```python
from build123d import *

# Parameters (mm, degrees)
SKETCH1_R           = 29
BOSS_EXTRUDE1_DEPTH = 30
SKETCH2_OUTSIDE_W   = 77.468
SKETCH2_OUTSIDE_H   = 77.468
SKETCH2_OUTSIDE_R   = 23
CUT_EXTRUDE1_DEPTH  = 22
CHAMFER1_SIZE       = 6
CHAMFER1_SIZE2      = 5.034597787
SKETCH3_R           = 25
BOSS_EXTRUDE2_DEPTH = 20
SKETCH4_R           = 5
BOSS_EXTRUDE3_DEPTH = 20
CHAMFER2_SIZE       = 2


with BuildPart() as part:
    # Sketch1 → Boss-Extrude1 (new body)
    with BuildSketch(Plane.XY):
        Circle(SKETCH1_R)
    extrude(amount=BOSS_EXTRUDE1_DEPTH)

    # Sketch2 outside → Cut-Extrude1 (cut)
    with BuildSketch(Plane.XY.offset(30)):
        Rectangle(SKETCH2_OUTSIDE_W, SKETCH2_OUTSIDE_H)
        Circle(SKETCH2_OUTSIDE_R, mode=Mode.SUBTRACT)
    extrude(amount=-CUT_EXTRUDE1_DEPTH, mode=Mode.SUBTRACT)

    # Chamfer1
    chamfer1_edges = [part.edges().sort_by_distance(p)[0] for p in [
        (-29, 0, 8),
    ]]
    chamfer1_side = [part.faces().sort_by_distance(p)[0] for p in [
        (-29, 0, 4),
    ]]
    chamfer(chamfer1_edges, length=CHAMFER1_SIZE, length2=CHAMFER1_SIZE2, reference=chamfer1_side[0])

    # Sketch3 → Boss-Extrude2 (add)
    with BuildSketch(Plane.XY.offset(30)):
        Circle(SKETCH3_R)
    extrude(amount=BOSS_EXTRUDE2_DEPTH)

    # Sketch4 → Boss-Extrude3 (add)
    with BuildSketch(Plane(origin=(0, 0, 0), x_dir=(-1, 0, 0), z_dir=(0, 0, -1))):
        Circle(SKETCH4_R)
    extrude(amount=BOSS_EXTRUDE3_DEPTH)

    # Chamfer2
    chamfer2_edges = [part.edges().sort_by_distance(p)[0] for p in [
        (-25, 0, 50),
    ]]
    chamfer(chamfer2_edges, length=CHAMFER2_SIZE)


solid = part.part
```
The model under review builds one solid part; all positions refer to its coordinate system, in mm. A direction names the side the tool comes from. Coordinates: 2 decimals unless noted, no trailing zeros. Order: outer loops, then holes, each group sorted by start corner. A loop starts at its lowest first (then second) coordinate and runs counter-clockwise, first axis right, second up. Notation, with made-up numbers: M 49.5,51.5 L 80.5,51.5 A23 ccw 80.5,88.5 Z; hole C -27.5,10 d9. An arc over 180 degrees is marked long. One line per question, with ' | ' between items.
(1) Add section D-D, the plane z = 45. Write out the cut boundary in (x, y), then the cut area to 3 significant figures.
Geometry results:
outline: C 0,0 d50 | area: 1,960 mm²
(2) For probe 1 along Z at (x, y) = (0, 24.5); probe 2 along Z at (x, y) = (-9, 9); probe 3 along Z at (x, y) = (12.5, -20), list the stretches that pass through material, from the lowest coordinate up. Write a range as from..to.
Geometry results:
probe 1: z = 0..7.36, 30..48.5 | probe 2: z = 0..50 | probe 3: z = 0..8, 30..49.42
(3) The part is to be moulded in two halves that separate along Z. For faces 4 (the face through (22.1, -7.3, 30)), 5 (the face through (1.08, -4.88, -9.86)), 6 (the face through (0, 0, -20)), say which applies: +Z half, -Z half, draft (parallel to the pull), parting line (faces both ways), or undercut.
Geometry results:
face 4: undercut | face 5: draft | face 6: -Z half
(4) Add section C-C, the plane z = -9. Write out the cut boundary in (x, y), then the cut area to 3 significant figures.
Geometry results:
outline: C 0,0 d10 | area: 78.5 mm²
(5) Insertion check: pin 1 (4 mm diameter, centred on x = -6.5, y = 23, fed in from +Z); pin 2 (12 mm diameter, centred on x = 3, z = 35.5, fed in from +Y); pin 3 (6 mm diameter, centred on x = -4, z = -7.5, fed in from -Y); pin 4 (1 mm diameter, centred on x = -9.5, z = 24.5, fed in from -Y). Each pin has a flat end and moves straight along its axis. Give the tip position at first contact, or say it passes through.
Geometry results:
pin 1: stops at z = 50 | pin 2: stops at y = 25 | pin 3: stops at y = -4.9 | pin 4: stops at y = -21.17
(6) Add section A-A, the plane y = 0. Write out the cut boundary in (x, z).
Geometry results:
outline: M -29,0 L -5,0 L -5,-20 L 5,-20 L 5,0 L 29,0 L 29,2 L 23.97,8 L 23,8 L 23,30 L 25,30 L 25,48 L 23,50 L -23,50 L -25,48 L -25,30 L -23,30 L -23,8 L -23.97,8 L -29,2 Z
(7) Machinability: for faces 1 (the face through (0, 0, 50)), 2 (the face through (23.846, 7.509, 38.874)), 3 (the face through (-5.25, 23.63, 7.71)), which of the approach directions +Z, -Z, +X, -X, +Y, -Y give a long, thin tool a straight path to every point of the face, cutting with its end or side? Answer none if there is none.
Geometry results:
face 1: +Z, +X, -X, +Y, -Y | face 2: +Z | face 3: none
